Design review of the part built by this model. Coordinates are the model's own, in mm. A direction names the side the tool comes from. Give positions to 0.01 mm unless a question says otherwise; leave off trailing zeros. Order: outer loops, then holes, each group sorted by start corner. A loop starts at its lowest first (then second) coordinate and runs counter-clockwise, first axis right, second up. Notation, with made-up numbers: (-38, 11.25) -> (17, 11.25) arc R18 ccw to (17, 37.25) -> close; hole circle Ø6 at (48.5, -16). An arc over 180 degrees is marked (long way). One line per item, written item: value.
from build123d import *

# Parameters (mm, degrees)
F0_W           = 133.35
F0_H           = 6.35
F1_DEPTH       = 283.464
F6_DEPTH       = 1.27
F7_D           = 5.1054
F7_CSINK_D     = 10.4394
F7_CSINK_ANGLE = 82
F9_D           = 5.1054
F9_CSINK_D     = 10.4394
F9_CSINK_ANGLE = 82
F11_DEPTH      = 6.351


with BuildPart() as f1:
    # F0 (on Top) → F1 (new body)
    with BuildSketch(Plane.XY):
        with Locations((66.675, 3.175)):
            Rectangle(F0_W, F0_H)
    extrude(amount=F1_DEPTH)

    # F5 (on face) → F6 (cut)
    with BuildSketch(Plane(origin=(0, 6.35, 0), x_dir=(-1, 0, 0), z_dir=(0, 1, 0))):
        with BuildLine():
            ThreePointArc((-102.87, 123.698), (-101.9400640303, 121.4529359697), (-99.695, 120.523))
            Line((-99.695, 120.523), (-75.080136745, 120.523))
            Line((-75.080136745, 120.523), (-58.2492406429, 103.6921038979))
            ThreePointArc((-58.2492406429, 103.6921038979), (-56.0041766126, 102.7621679282), (-53.7591125824, 103.6921038979))
            Line((-53.7591125824, 103.6921038979), (-36.9282164803, 120.523))
            Line((-36.9282164803, 120.523), (-33.655, 120.523))
            ThreePointArc((-33.655, 120.523), (-31.4099359697, 121.4529359697), (-30.48, 123.698))
            Line((-30.48, 123.698), (-30.48, 126.9712164803))
            Line((-30.48, 126.9712164803), (-28.2551851985, 129.1960312817))
            ThreePointArc((-28.2551851985, 129.1960312817), (-27.3252492288, 131.441095312), (-28.2551851985, 133.6861593423))
            Line((-28.2551851985, 133.6861593423), (-30.48, 135.9109741438))
            Line((-30.48, 135.9109741438), (-30.48, 159.766))
            ThreePointArc((-30.48, 159.766), (-31.4099359697, 162.0110640303), (-33.655, 162.941))
            Line((-33.655, 162.941), (-57.5100258562, 162.941))
            Line((-57.5100258562, 162.941), (-74.9525170281, 180.3834911718))
            ThreePointArc((-74.9525170281, 180.3834911718), (-77.1975810584, 181.3134271416), (-79.4426450886, 180.3834911718))
            Line((-79.4426450886, 180.3834911718), (-96.8851362605, 162.941))
            Line((-96.8851362605, 162.941), (-99.695, 162.941))
            ThreePointArc((-99.695, 162.941), (-101.9400640303, 162.0110640303), (-102.87, 159.766))
            Line((-102.87, 159.766), (-102.87, 156.9561362605))
            Line((-102.87, 156.9561362605), (-104.9465724725, 154.879563788))
            ThreePointArc((-104.9465724725, 154.879563788), (-105.8765084422, 152.6344997577), (-104.9465724725, 150.3894357275))
            Line((-104.9465724725, 150.3894357275), (-102.87, 148.312863255))
            Line((-102.87, 148.312863255), (-102.87, 123.698))
        make_face()
    extrude(amount=-F6_DEPTH, mode=Mode.SUBTRACT)

    # F7 (through all)
    with Locations(Plane.XZ):
        with Locations((39.65575, 141.732), (93.69425, 141.732), (85.7804948976, 160.8374948976), (47.5695051024, 122.6265051024)):
            CounterSinkHole(F7_D / 2, F7_CSINK_D / 2, counter_sink_angle=F7_CSINK_ANGLE)

    # F9 (through all)
    with Locations(Plane(origin=(0, 6.35, 0), x_dir=(-1, 0, 0), z_dir=(0, 1, 0))):
        with Locations((-22.225, 271.907), (-111.125, 271.907), (-22.225, 11.557), (-111.125, 11.557), (-111.125, 240.411), (-22.225, 240.411), (-111.125, 43.053), (-22.225, 43.053)):
            CounterSinkHole(F9_D / 2, F9_CSINK_D / 2, counter_sink_angle=F9_CSINK_ANGLE)

    # F10 (on face) → F11 (cut, through all)
    with BuildSketch(Plane.XZ):
        with BuildLine():
            ThreePointArc((78.105, 175.2607215967), (79.8985168363, 181.7675353331), (84.7725, 186.4365411975))
            ThreePointArc((84.7725, 186.4365411975), (66.675, 258.064), (48.5775, 186.4365411975))
            ThreePointArc((48.5775, 186.4365411975), (53.4514831637, 181.7675353331), (55.245, 175.2607215967))
            Line((55.245, 175.2607215967), (55.245, 108.2032784033))
            ThreePointArc((55.245, 108.2032784033), (53.4514831637, 101.6964646669), (48.5775, 97.0274588025))
            ThreePointArc((48.5775, 97.0274588025), (66.675, 25.4), (84.7725, 97.0274588025))
            ThreePointArc((84.7725, 97.0274588025), (79.8985168363, 101.6964646669), (78.105, 108.2032784033))
            Line((78.105, 108.2032784033), (78.105, 175.2607215967))
        make_face()
    extrude(amount=-F11_DEPTH, mode=Mode.SUBTRACT)


solid = f1.part
Item 1: Add section B-B on x = 72.5. Give the boundary of the cut face in (y, z), plus the area to 3 significant figures.
Returned:
outline: (0, 0) -> (6.35, 0) -> (6.35, 25.85) -> (0, 25.85) -> close; (0, 257.62) -> (6.35, 257.62) -> (6.35, 283.46) -> (0, 283.46) -> close
area: 328 mm²
Item 2: Machinability: for faces 4 (the flat face through (78.105, 2, 141)), 5 (the conical face through (112.567, 3.431, 13.819)), which of the approach directions +Z, -Z, +X, -X, +Y, -Y give a long, thin tool a straight path to every point of the face, cutting with its end or side? Answer none if there is none.
Returned:
face 4: +Y, -Y
face 5: +Y
Item 3: To check wall thickness, follow line 1 along X through (y, z) = (6.25, 16); line 2 along X through (y, z) = (2, 63.5) (3 decimals); line 3 along X through (y, z) = (1, 148) (3 decimals). State the ranges of each line that lie inside material, in increasing order. Write a range as from..to.
Returned:
line 1: 0..19.65, 24.8..108.55, 113.7..133.35
line 2: 0..28.575, 104.775..133.35
line 3: 0..55.245, 78.105..133.35
Item 4: Draft analysis for pull direction Y (two halves, no side actions). For faces 1 (the conical face through (87.76, 2.92, 162.65)), 2 (the cylindrical face through (68.086, 3.131, 258.038)), 3 (the conical face through (112.567, 3.431, 274.169)), state which applies: pulls with the +Y half, pulls with the -Y half, needs draft (parallel to the pull), parting line crosses it, or undercut.
Returned:
face 1: pulls with the -Y half
face 2: needs draft
face 3: pulls with the +Y half
Item 5: Add section A-A on z = 63.5. Give the boundary of the cut face in (x, y) (3 decimals), plus the area to 3 significant figures.
Returned:
outline: (0, 0) -> (28.575, 0) -> (28.575, 6.35) -> (0, 6.35) -> close; (104.775, 0) -> (133.35, 0) -> (133.35, 6.35) -> (104.775, 6.35) -> close
area: 363 mm²
Item 6: Clearance check with a flat-ended pin moving along its axis: P1, Ø1.4, axis at y = 5.5, z = 158, coming from the -X side. State where the tip first meets the part, or that it passes through.
Returned:
P1: x = 0
